CAD build for the part. Positions are in the model's coordinates, mm. Face numbers are marked on the shaded views. A direction names the side the tool comes from. Round coordinates to 2 decimals unless told otherwise and drop trailing zeros. Loops run counter-clockwise (first coordinate to the right, second up) from the corner with the lowest first, then second, coordinate; pieces in that order, holes last. Notation, with made-up numbers: M 82,50 L 121,50 A19 ccw 121,76 Z; hole C 1,-26 d9. An arc over 180 degrees is marked long. One line per item, written item: value. Start each with the question number.
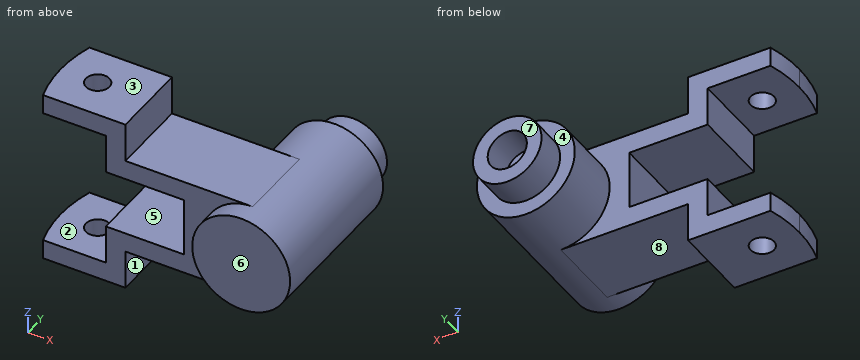
from build123d import *

# Parameters (mm, degrees)
BOSS_EXTRUDE1_DEPTH     = 40
CUT_EXTRUDE2_DEPTH      = 90
CUT_EXTRUDE4_DEPTH      = 151
CUT_EXTRUDE4_DEPTH_BACK = 151
SKETCH3_R               = 6
BOSS_EXTRUDE2_START     = -10
BOSS_EXTRUDE2_OUTLINE_R = 25
BOSS_EXTRUDE2_DEPTH     = 80
SKETCH5_R               = 17.5
SKETCH5_R_2             = 10
BOSS_EXTRUDE3_DEPTH     = 86


# Read off the part's stored shape, not the designer's step: Boss-Extrude2
with BuildPart() as part:
    # Sketch1 → Boss-Extrude1 (new body)
    with BuildSketch(Plane(origin=(0, 0, 0), x_dir=(1, 0, 0), z_dir=(0, 1, 0))):
        Polygon((-56.273517373, 36.016865909), (-56.273517373, 26.016865909), (-21.273517373, 26.016865909), (-21.273517373, 6.016865909), (18.726482627, 6.016865909), (18.726482627, -23.983134091), (-21.273517373, -23.983134091), (-21.273517373, -43.983134091), (-56.273517373, -43.983134091), (-56.273517373, -53.983134091), (-11.273517373, -53.983134091), (-11.273517373, -33.983134091), (53.726482627, -33.983134091), (53.726482627, 16.016865909), (-11.273517373, 16.016865909), (-11.273517373, 36.016865909), align=None)
    extrude(amount=BOSS_EXTRUDE1_DEPTH)

    # Sketch2 → Cut-Extrude2 (cut)
    with BuildSketch(Plane.XY.offset(53.983134091)):
        with BuildLine():
            ThreePointArc((-53.355556698, 0), (-55.540185955, 9.89412925), (-56.273517373, 20))
            Line((-56.273517373, 20), (-56.273517373, 0))
            Line((-56.273517373, 0), (-53.355556698, 0))
        make_face()
        with BuildLine():
            ThreePointArc((-56.273517373, 20), (-55.540185955, 30.10587075), (-53.355556698, 40))
            Line((-53.355556698, 40), (-56.273517373, 40))
            Line((-56.273517373, 40), (-56.273517373, 20))
        make_face()
    extrude(amount=-CUT_EXTRUDE2_DEPTH, mode=Mode.SUBTRACT)

    # Sketch3 → Cut-Extrude4 (cut, two sides: drawn at the far end of the back side and taken through both)
    with BuildSketch(Plane.XY.offset(-26.016865909).offset(-CUT_EXTRUDE4_DEPTH_BACK)):
        with Locations(Location((-37.314537036, 20, 0), (0, 0, 180))):
            Circle(SKETCH3_R)
    extrude(amount=CUT_EXTRUDE4_DEPTH + CUT_EXTRUDE4_DEPTH_BACK, mode=Mode.SUBTRACT)

    # Boss-Extrude2 outline → Boss-Extrude2 (add)
    with BuildSketch(Plane(origin=(0, 0, 0), x_dir=(1, 0, 0), z_dir=(0, 1, 0)).offset(BOSS_EXTRUDE2_START)):
        with Locations((53.726482627, -8.983134091)):
            Circle(BOSS_EXTRUDE2_OUTLINE_R)
    extrude(amount=BOSS_EXTRUDE2_DEPTH)

    # Sketch5 → Boss-Extrude3 (add)
    with BuildSketch(Plane(origin=(0, 0, 0), x_dir=(1, 0, 0), z_dir=(0, 1, 0))):
        with Locations(Location((53.726482627, -8.983134091, 0), (0, 0, 270))):
            Circle(SKETCH5_R)
        with Locations(Location((53.726482627, -8.983134091, 0), (0, 0, 270))):
            Circle(SKETCH5_R_2, mode=Mode.SUBTRACT)
    extrude(amount=BOSS_EXTRUDE3_DEPTH)


solid = part.part
(1) Flat gauge pins, fed straight in: P1, Ø12, axis at x = -7, y = 15, coming from the -Z side; P2, Ø20, axis at x = 30.5, y = 28, coming from the +Z side; P3, Ø1.5, axis at y = 23.5, z = 1.5, coming from the +X side; P4, Ø5, axis at x = 35, y = 60, coming from the +Z side. Where does each tip first touch, or does it go through?
(2) Probe L1, parallel to X at y = 77.5, z = 9; L2, parallel to Z at x = -32, y = 33.5; L3, parallel to Z at x = -3.5, y = 17.5. List the from-to ranges inside material, lowest first.
(3) Mould opens along Z. For the marked faces 1, 2 and 3 say: pulls with the +Z half, pulls with the -Z half, needs draft (parallel to the pull), parting line crosses it, or undercut.
(4) Which spindle directions (+Z, -Z, +X, -X, +Y, -Y) get a long thin tool onto all of the face, cutting with end or side? Do the marked faces 4, 5, 6, 7 and 8. Say none if no direction does.
(5) Slice it at A-A, the plane y = 76. List the corners of the cut face in (x, z).
(6) Slice it at D-D, the plane x = 24.5. List the corners of the cut face in (y, z), and give its area (3 significant figures).
(7) Slice it at C-C, the plane y = 3. List the corners of the cut face in (x, z).
(8) Slice it at B-B, the plane z = -13.5. List the corners of the cut face in (x, y).
Check result:
1. P1: stops at z = -36.02
1. P2: stops at z = 33.98
1. P3: stops at x = 77.8
1. P4: stops at z = 28
2. L1: x = 36.23 to 43.73, 63.73 to 71.23
2. L2: z = -36.02 to -26.02, 43.98 to 53.98
2. L3: z = -16.02 to -6.02, 23.98 to 33.98
3. face 1: needs draft
3. face 2: undercut
3. face 3: pulls with the +Z half
4. face 4: +Y
4. face 5: -X, +Y, -Y
4. face 6: +Z, -Z, +X, -X, -Y
4. face 7: +Z, -Z, +X, -X, +Y
4. face 8: -Z, +X, +Y, -Y
5. outline: C 53.73,8.98 d35; hole C 53.73,8.98 d20
6. outline: M 0,-16.02 L 40,-16.02 L 40,33.98 L 0,33.98 Z
6. area: 2,000 mm^2
7. outline: M -54.18,-36.02 L -11.27,-36.02 L -11.27,-16.02 L 53.73,-16.02 A25 ccw 53.73,33.98 L -11.27,33.98 L -11.27,53.98 L -54.18,53.98 L -54.18,43.98 L -21.27,43.98 L -21.27,23.98 L 18.73,23.98 L 18.73,-6.02 L -21.27,-6.02 L -21.27,-26.02 L -54.18,-26.02 Z
8. outline: M -21.27,0 L 42.79,0 L 42.79,-10 L 64.66,-10 L 64.66,70 L 42.79,70 L 42.79,40 L -21.27,40 Z
